```python
from build123d import *

# Parameters (mm, degrees)
SKETCH1_W                = 20
SKETCH1_H                = 50.5
BOSS_EXTRUDE1_DEPTH      = 7.5
SKETCH2_W                = 20
SKETCH2_H                = 10
BOSS_EXTRUDE2_DEPTH      = 14.01
LPATTERN1_COUNT          = 7
LPATTERN1_PITCH          = 40
SKETCH4_W                = 40.5
SKETCH4_H                = 7.5
BOSS_EXTRUDE3_DEPTH      = 260
M4_CLEARANCE_HOLE1_D     = 4.5
M4_CLEARANCE_HOLE1_DEPTH = 7.5
LPATTERN2_COUNT          = 7
LPATTERN2_PITCH          = 40
SKETCH7_W                = 18
SKETCH7_H                = 18
CUT_EXTRUDE1_DEPTH       = 8.5
FILLET1_R                = 2
LPATTERN3_COUNT          = 6
LPATTERN3_PITCH          = 40
FILLET1_OF_LPATTERN3_R   = 2
FILLET2_R                = 5
CHAMFER1_SIZE            = 2
CHAMFER2_SIZE            = 2


with BuildPart() as part:
    # Sketch1 → Boss-Extrude1 (new body)
    with BuildSketch(Plane(origin=(0, 0, 0), x_dir=(1, 0, 0), z_dir=(0, 1, 0))):
        with Locations((0, -25.25)):
            Rectangle(SKETCH1_W, SKETCH1_H)
    extrude(amount=BOSS_EXTRUDE1_DEPTH)

    # Sketch2 → Boss-Extrude2 (add)
    with BuildSketch(Plane(origin=(0, 7.5, 0), x_dir=(1, 0, 0), z_dir=(0, 1, 0))):
        with Locations((0, -45.5)):
            Rectangle(SKETCH2_W, SKETCH2_H)
    extrude(amount=BOSS_EXTRUDE2_DEPTH)


with BuildPart() as lpattern1_1:
    # LPattern1: pattern copy
    add(part.part.moved(Location(Vector(1, 0, 0) * (1 * LPATTERN1_PITCH))))


with BuildPart() as lpattern1_2:
    # LPattern1: pattern copy
    add(part.part.moved(Location(Vector(1, 0, 0) * (2 * LPATTERN1_PITCH))))


with BuildPart() as lpattern1_3:
    # LPattern1: pattern copy
    add(part.part.moved(Location(Vector(1, 0, 0) * (3 * LPATTERN1_PITCH))))


with BuildPart() as lpattern1_4:
    # LPattern1: pattern copy
    add(part.part.moved(Location(Vector(1, 0, 0) * (4 * LPATTERN1_PITCH))))


with BuildPart() as lpattern1_5:
    # LPattern1: pattern copy
    add(part.part.moved(Location(Vector(1, 0, 0) * (5 * LPATTERN1_PITCH))))


with BuildPart() as lpattern1_6:
    # LPattern1: pattern copy
    add(part.part.moved(Location(Vector(1, 0, 0) * (6 * LPATTERN1_PITCH))))


with BuildPart() as part_1:
    add(part.part)

    add(lpattern1_1.part)  # Boss-Extrude3 merges LPattern1_1

    add(lpattern1_2.part)  # Boss-Extrude3 merges LPattern1_2

    add(lpattern1_3.part)  # Boss-Extrude3 merges LPattern1_3

    add(lpattern1_4.part)  # Boss-Extrude3 merges LPattern1_4

    add(lpattern1_5.part)  # Boss-Extrude3 merges LPattern1_5

    add(lpattern1_6.part)  # Boss-Extrude3 merges LPattern1_6
    # Sketch4 → Boss-Extrude3 (add, through all)
    with BuildSketch(Plane.ZY.offset(10)):
        with Locations((20.25, 3.75)):
            Rectangle(SKETCH4_W, SKETCH4_H)
    extrude(amount=-BOSS_EXTRUDE3_DEPTH)

    # M4 Clearance Hole1
    with Locations(Plane.XZ):
        with Locations((240, 20)):
            m4_clearance_hole1 = Hole(M4_CLEARANCE_HOLE1_D / 2, depth=M4_CLEARANCE_HOLE1_DEPTH)

    # LPattern2: M4 Clearance Hole1 ×7
    with Locations(*[(-i * LPATTERN2_PITCH, 0, 0) for i in range(1, LPATTERN2_COUNT)]):
        add(m4_clearance_hole1, mode=Mode.SUBTRACT)

    # Sketch7 → Cut-Extrude1 (cut, through all)
    with BuildSketch(Plane(origin=(0, 7.5, 0), x_dir=(1, 0, 0), z_dir=(0, 1, 0))):
        with Locations((220, -20.25)):
            Rectangle(SKETCH7_W, SKETCH7_H)
    cut_extrude1 = extrude(amount=-CUT_EXTRUDE1_DEPTH, mode=Mode.SUBTRACT)

    # Fillet1
    fillet1_edges = [part_1.edges().sort_by_distance(p)[0] for p in [
        (229, 3.75, 11.25),
        (229, 3.75, 29.25),
        (211, 3.75, 29.25),
        (211, 3.75, 11.25),
    ]]
    fillet(fillet1_edges, radius=FILLET1_R)

    # LPattern3: Cut-Extrude1 ×6
    with Locations(*[(-i * LPATTERN3_PITCH, 0, 0) for i in range(1, LPATTERN3_COUNT)]):
        add(cut_extrude1, mode=Mode.SUBTRACT)

    # Fillet1 of LPattern3
    fillet1_of_lpattern3_edges = [part_1.edges().sort_by_distance(p)[0] for p in [
        (189, 3.75, 11.25),
        (189, 3.75, 29.25),
        (171, 3.75, 29.25),
        (171, 3.75, 11.25),
        (149, 3.75, 11.25),
        (149, 3.75, 29.25),
        (131, 3.75, 29.25),
        (131, 3.75, 11.25),
        (109, 3.75, 11.25),
        (109, 3.75, 29.25),
        (91, 3.75, 29.25),
        (91, 3.75, 11.25),
        (69, 3.75, 11.25),
        (69, 3.75, 29.25),
        (51, 3.75, 29.25),
        (51, 3.75, 11.25),
        (29, 3.75, 11.25),
        (29, 3.75, 29.25),
        (11, 3.75, 29.25),
        (11, 3.75, 11.25),
    ]]
    fillet(fillet1_of_lpattern3_edges, radius=FILLET1_OF_LPATTERN3_R)

    # Fillet2
    fillet2_edges = [part_1.edges().sort_by_distance(p)[0] for p in [
        (250, 3.75, 0),
        (-10, 3.75, 0),
    ]]
    fillet(fillet2_edges, radius=FILLET2_R)

    # Chamfer1
    chamfer1_edges = [part_1.edges().sort_by_distance(p)[0] for p in [
        (120, 21.51, 50.5),
        (160, 21.51, 50.5),
        (200, 21.51, 50.5),
        (240, 21.51, 50.5),
        (0, 21.51, 50.5),
        (40, 21.51, 50.5),
        (80, 21.51, 50.5),
    ]]
    chamfer(chamfer1_edges, length=CHAMFER1_SIZE)

    # Chamfer2
    chamfer2_edges = [part_1.edges().sort_by_distance(p)[0] for p in [
        (110, 3.75, 40.5),
        (130, 3.75, 40.5),
        (150, 3.75, 40.5),
        (170, 3.75, 40.5),
        (190, 3.75, 40.5),
        (210, 3.75, 40.5),
        (230, 3.75, 40.5),
        (10, 3.75, 40.5),
        (50, 3.75, 40.5),
        (30, 3.75, 40.5),
        (70, 3.75, 40.5),
        (90, 3.75, 40.5),
    ]]
    chamfer(chamfer2_edges, length=CHAMFER2_SIZE)


solid = part_1.part
```
Can you work these out from the model? Positions are in its coordinate system, mm. A direction names the side the tool comes from. Coordinates: 2 decimals unless noted, no trailing zeros. Loops run counter-clockwise (first coordinate to the right, second up) from the corner with the lowest first, then second, coordinate; pieces in that order, holes last. Notation, with made-up numbers: (27.25, 85) - (39.25, 85) arc R27 cw to (39.25, 118) - close; hole circle Ø10 at (-32, -22.75). An arc over 180 degrees is marked (long way). Use a Markdown table: item, result.
Item 1: We'd pull the mould along X, two halves only. Please class faces 4 (the face through (117.92, 3.8, 19.14)), 5 (the face through (-10, 6, 33)), 6 (the face through (160, 10, 50.5)): released by +X, released by -X, zero draft, split by the parting line, or undercut.
Numbers:
| item | result |
|---|---|
| face 4 | undercut |
| face 5 | released by -X |
| face 6 | zero draft |
Item 2: I want a section at C-C on y = 15. Please give me the cut outline in (x, z), and give its area (3 significant figures).
Numbers:
| item | result |
|---|---|
| outline | (-10, 40.5) - (10, 40.5) - (10, 50.5) - (-10, 50.5) - close; (30, 40.5) - (50, 40.5) - (50, 50.5) - (30, 50.5) - close; (70, 40.5) - (90, 40.5) - (90, 50.5) - (70, 50.5) - close; (110, 40.5) - (130, 40.5) - (130, 50.5) - (110, 50.5) - close; (150, 40.5) - (170, 40.5) - (170, 50.5) - (150, 50.5) - close; (190, 40.5) - (210, 40.5) - (210, 50.5) - (190, 50.5) - close; (230, 40.5) - (250, 40.5) - (250, 50.5) - (230, 50.5) - close |
| area | 1,400 mm2 |
Item 3: For faces 1 (the face through (0, 14, 40.5)), 2 (the face through (100, 4, 40.5)), 3 (the face through (211, 4, 20)), which set-ups out of +Z, -Z, +X, -X, +Y, -Y let a thin tool reach every point of the face, with its end or its side?
Numbers:
| item | result |
|---|---|
| face 1 | -Z, +X, -X, +Y |
| face 2 | +Z, +Y, -Y |
| face 3 | +Y, -Y |
Item 4: I want a section at A-A on z = 25. Please give me the cut outline in (x, y).
Numbers:
| item | result |
|---|---|
| outline | (-10, 0) - (11, 0) - (11, 7.5) - (-10, 7.5) - close; (29, 0) - (51, 0) - (51, 7.5) - (29, 7.5) - close; (69, 0) - (91, 0) - (91, 7.5) - (69, 7.5) - close; (109, 0) - (131, 0) - (131, 7.5) - (109, 7.5) - close; (149, 0) - (171, 0) - (171, 7.5) - (149, 7.5) - close; (189, 0) - (211, 0) - (211, 7.5) - (189, 7.5) - close; (229, 0) - (250, 0) - (250, 7.5) - (229, 7.5) - close |
Item 5: I want a section at B-B on x = 40. Please give me the cut outline in (y, z).
Numbers:
| item | result |
|---|---|
| outline | (0, 0) - (7.5, 0) - (7.5, 17.75) - (0, 17.75) - close; (0, 22.25) - (7.5, 22.25) - (7.5, 40.5) - (21.51, 40.5) - (21.51, 48.5) - (19.51, 50.5) - (0, 50.5) - close |
Item 6: I want a section at D-D on x = 181.5. Please give me the cut outline in (y, z).
Numbers:
| item | result |
|---|---|
| outline | (0, 0) - (7.5, 0) - (7.5, 11.25) - (0, 11.25) - close; (0, 29.25) - (7.5, 29.25) - (7.5, 40.5) - (0, 40.5) - close |
Item 7: Will these pins go through, and if not, where does the flat tip stop? pin 1 (7 mm diameter, centred on x = 160, z = 20, fed in from +Y); pin 2 (1 mm diameter, centred on x = 188, y = 15.5, fed in from +Z); pin 3 (7 mm diameter, centred on x = 116, y = 15, fed in from -Z); pin 4 (2 mm diameter, centred on x = 62.5, y = 3.5, fed in from +Z).
Numbers:
| item | result |
|---|---|
| pin 1 | stops at y = 7.5 |
| pin 2 | passes through |
| pin 3 | stops at z = 40.5 |
| pin 4 | stops at z = 40.5 |
Item 8: If I drill on probe 1 along Z at (x, y) = (62.5, 4.25); probe 2 along Y at (x, z) = (187.5, 36); probe 3 along Z at (x, y) = (230.5, 17.75), over which ranges is the centre line in solid material (lowest first)? Write a range as from..to.
Numbers:
| item | result |
|---|---|
| probe 1 | z = 0..11.25, 29.25..40.5 |
| probe 2 | y = 0..7.5 |
| probe 3 | z = 40.5..50.5 |
